The listing builds one solid part. Answer for the finished solid, in the listing's coordinates (mm). Face numbers are marked on the shaded views. A direction names the side the tool comes from. Give positions to 0.01 mm unless a question says otherwise; leave off trailing zeros. Order: outer loops, then holes, each group sorted by start corner. A loop starts at its lowest first (then second) coordinate and runs counter-clockwise, first axis right, second up. Notation, with made-up numbers: (79.5, -31.75) - (95.5, -31.75) arc R19 cw to (95.5, -20.75) - close; hole circle Ø11 at (38, 49). An arc over 180 degrees is marked (long way). Answer in a Markdown table with one row per item.
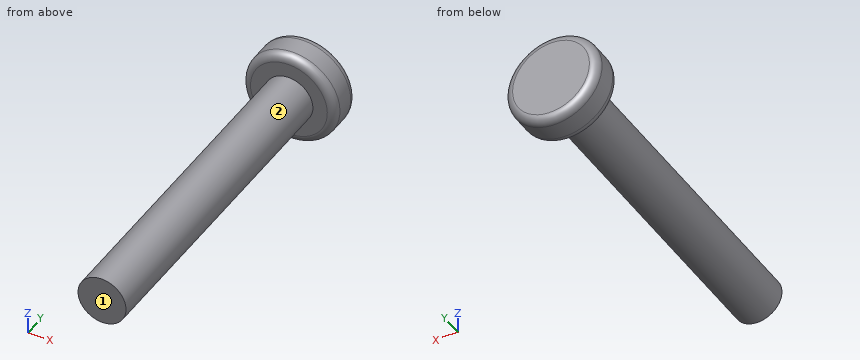
from build123d import *

# Parameters (mm, degrees)
SKETCH1_R           = 3
BOSS_EXTRUDE1_DEPTH = 40
SKETCH2_R           = 5.8
BOSS_EXTRUDE2_DEPTH = 4.3
FILLET1_R           = 1


with BuildPart() as part:
    # Sketch1 → Boss-Extrude1 (new body)
    with BuildSketch(Plane(origin=(0, 0, 0), x_dir=(1, 0, 0), z_dir=(0, 1, 0))):
        with Locations(Location((0, 0, 0), (0, 0, 270))):  # turned: the seam where the file's is
            Circle(SKETCH1_R)
    extrude(amount=BOSS_EXTRUDE1_DEPTH)

    # Sketch2 → Boss-Extrude2 (add)
    with BuildSketch(Plane(origin=(0, 40, 0), x_dir=(1, 0, 0), z_dir=(0, 1, 0))):
        with Locations(Location((0, 0, 0), (0, 0, 270))):  # turned: the seam where the file's is
            Circle(SKETCH2_R)
    extrude(amount=BOSS_EXTRUDE2_DEPTH)

    # Fillet1
    fillet1_edges = [part.edges().sort_by_distance(p)[0] for p in [
        (0, 40, -5.8),
        (0, 44.3, -5.8),
    ]]
    fillet(fillet1_edges, radius=FILLET1_R)


solid = part.part
Item 1: Find section C-C on y = 17. Write down the section's boundary in (x, z).
Answer block:
| item | result |
|---|---|
| outline | circle Ø6 at (0, 0) |
Item 2: Consider line 1 (Y direction, x = -2, z = 3.5); line 2 (Z direction, x = -0.25, y = 27.5); line 3 (Z direction, x = -1.5, y = 27.5). Determine where each line is inside the solid, lowest interval first.
Answer block:
| item | result |
|---|---|
| line 1 | 40 to 44.3 |
| line 2 | -2.99 to 2.99 |
| line 3 | -2.6 to 2.6 |
Item 3: Find section A-A on z = 0. Write down the section's boundary in (x, y), then the cut area to 3 significant figures.
Answer block:
| item | result |
|---|---|
| outline | (-5.8, 41) arc R1 ccw to (-4.8, 40) - (-3, 40) - (-3, 0) - (3, 0) - (3, 40) - (4.8, 40) arc R1 ccw to (5.8, 41) - (5.8, 43.3) arc R1 ccw to (4.8, 44.3) - (-4.8, 44.3) arc R1 ccw to (-5.8, 43.3) - close |
| area | 289 mm² |
Item 4: Each of these flat-tipped pins is pushed along its axis until it touches: P1, Ø3, axis at y = 29.5, z = 1.5, coming from the +X side; P2, Ø1.5, axis at x = 3.5, y = 15, coming from the +Z side; P3, Ø6, axis at x = 0, y = 8.5, coming from the -Z side. Where does it stop, or does it pass through?
Answer block:
| item | result |
|---|---|
| P1 | x = 3 |
| P2 | z = 1.2 |
| P3 | z = -3 |
Item 5: Find section B-B on x = 0. Write down the section's boundary in (y, z), then the cut area to 3 significant figures.
Answer block:
| item | result |
|---|---|
| outline | (0, -3) - (40, -3) - (40, -4.8) arc R1 ccw to (41, -5.8) - (43.3, -5.8) arc R1 ccw to (44.3, -4.8) - (44.3, 4.8) arc R1 ccw to (43.3, 5.8) - (41, 5.8) arc R1 ccw to (40, 4.8) - (40, 3) - (0, 3) - close |
| area | 289 mm² |
Item 6: Which of the six approach directions +Z, -Z, +X, -X, +Y, -Y give full straight-line access (tool end or side, diameter ignored) to the marked faces 1 and 2?
Answer block:
| item | result |
|---|---|
| face 1 | +Z, -Z, +X, -X, -Y |
| face 2 | -Y |
